Verification items for the finished model (mm, model axes). Face numbers are marked on the shaded views. A direction names the side the tool comes from. Coordinates: 2 decimals unless noted, no trailing zeros. Order: outer loops, then holes, each group sorted by start corner. A loop starts at its lowest first (then second) coordinate and runs counter-clockwise, first axis right, second up. Notation, with made-up numbers: M -10.75,71 L 13.25,71 A22 cw 13.25,82 Z; hole C 86.5,-4 d7. An arc over 180 degrees is marked long. Answer as a JSON object with one key per item and string values. Group by question number.
(1) Mould release check, pull along Y, two halves, no side actions. Record for the marked faces 3, 4 and 5: released by +Y, released by -Y, zero draft, split by the parting line, or undercut.
(2) Gauge pin test, flat ends, axial feed: pin 1 Ø1 at (x, y) = (-3.5, -28) entering from +Z; pin 2 Ø1.5 at (x, z) = (-74.39, -4.15) entering from +Y; pin 3 Ø2 at (x, y) = (-25, -27) entering from -Z. Record the tip position at first contact, or that the pin passes through.
(3) Cross-section at A-A (z = -13). Enter the section's corners in (x, y), plus the area to 3 significant figures.
(4) Material ranges on line 1 (X direction, y = -35, z = -4.15); line 2 (X direction, y = -31.5, z = -13); line 3 (Y direction, x = -78, z = -18), recorded low to high.
(5) Cross-section at C-C (y = -35.75). Count the separate pieces of the cut face and the enclosed holes in it, plus the area to 3 significant figures.
(6) Cross-section at D-D (x = -32.5). Enter the section's corners in (y, z), plus the area to 3 significant figures.
(7) Access from +Z, -Z, +X, -X, +Y, -Y to the whole of each face (thin tool, end or side, straight path). Record for the marked faces 1 and 2.
(8) Cross-section at B-B (z = -19.25). Enter the section's corners in (x, y).
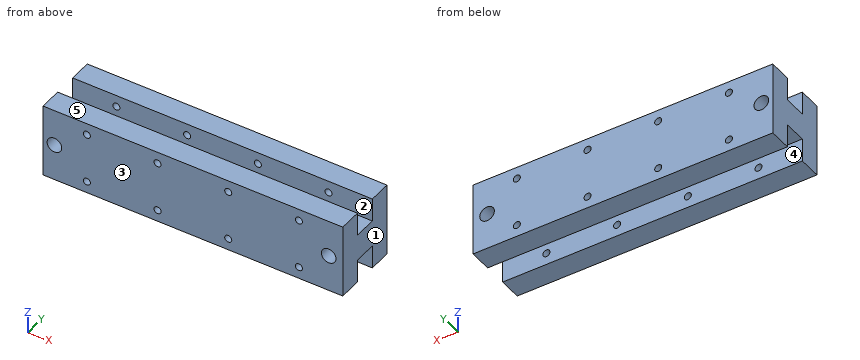
from build123d import *

# Parameters (mm, degrees)
SKETCH4_W                  = 106
SKETCH4_H                  = 24
BOSS_EXTRUDE2_DEPTH        = 13
CUT_EXTRUDE3_START         = -8.3
SKETCH25_W                 = 106
SKETCH25_H                 = 8.1
CUT_EXTRUDE3_DEPTH         = 108.807903902
M3X0_5_TAPPED_HOLE1_D      = 2.5
MIRROR3_START              = -40.65
MIRROR3_OUTLINE_W          = 106
MIRROR3_OUTLINE_H          = 4.7
MIRROR3_DEPTH              = 24
MIRROR3_START_2            = -24.601316976
MIRROR3_2_OUTLINE_W        = 106
MIRROR3_2_OUTLINE_H        = 8.3
MIRROR3_2_OUTLINE_R        = 1.25
MIRROR3_2_DEPTH            = 7.951316976
MIRROR3_3_OUTLINE_W        = 106
MIRROR3_3_OUTLINE_H        = 8.3
MIRROR3_3_OUTLINE_R        = 1.25
MIRROR3_3_DEPTH            = 7.948683024
F_6_0_204_DIAMETER_HOLE1_D = 5.1816


# Read off the part's stored shape, not the designer's step: Mirror3
with BuildPart() as part:
    # Sketch4 → Boss-Extrude2 (new body)
    with BuildSketch(Plane.XY):
        with Locations((-36.891047602, -28.65)):
            Rectangle(SKETCH4_W, SKETCH4_H)
    extrude(amount=-BOSS_EXTRUDE2_DEPTH)

    # Sketch25 → Cut-Extrude3 (cut)
    with BuildSketch(Plane.XY.offset(CUT_EXTRUDE3_START)):
        with Locations((-36.891047602, -28.651316976)):
            Rectangle(SKETCH25_W, SKETCH25_H)
    extrude(amount=CUT_EXTRUDE3_DEPTH, mode=Mode.SUBTRACT)

    # M3x0.5 Tapped Hole1 (through all)
    with Locations(Plane(origin=(-74.390985602, -16.65, -4.15), x_dir=(0, 0, 1), z_dir=(0, 1, 0))):
        with Locations((0, 0), (0, 25), (-0.055677319, 74.999938), (0, 50)):
            Hole(M3X0_5_TAPPED_HOLE1_D / 2)

    # Mirror3 outline → Mirror3 (add)
    with BuildSketch(Plane(origin=(0, 0, 0), x_dir=(1, 0, 0), z_dir=(0, 1, 0)).offset(MIRROR3_START)):
        with Locations((-36.891047602, 15.35)):
            Rectangle(MIRROR3_OUTLINE_W, MIRROR3_OUTLINE_H)
    extrude(amount=MIRROR3_DEPTH)

    # Mirror3 2 outline → Mirror3 2 (add)
    with BuildSketch(Plane(origin=(0, 0, 0), x_dir=(1, 0, 0), z_dir=(0, 1, 0)).offset(MIRROR3_START_2)):
        with Locations((-36.891047602, 21.85)):
            Rectangle(MIRROR3_2_OUTLINE_W, MIRROR3_2_OUTLINE_H)
        with Locations((-74.390985602, 21.85)):
            Circle(MIRROR3_2_OUTLINE_R, mode=Mode.SUBTRACT)
        with Locations((-49.390985602, 21.85)):
            Circle(MIRROR3_2_OUTLINE_R, mode=Mode.SUBTRACT)
        with Locations((-24.390985602, 21.85)):
            Circle(MIRROR3_2_OUTLINE_R, mode=Mode.SUBTRACT)
        with Locations((0.608952398, 21.794322681)):
            Circle(MIRROR3_2_OUTLINE_R, mode=Mode.SUBTRACT)
    extrude(amount=MIRROR3_2_DEPTH)

    # Mirror3 3 outline → Mirror3 3 (add)
    with BuildSketch(Plane(origin=(0, 0, 0), x_dir=(1, 0, 0), z_dir=(0, 1, 0)).offset(MIRROR3_START)):
        with Locations((-36.891047602, 21.85)):
            Rectangle(MIRROR3_3_OUTLINE_W, MIRROR3_3_OUTLINE_H)
        with Locations((-74.390985602, 21.85)):
            Circle(MIRROR3_3_OUTLINE_R, mode=Mode.SUBTRACT)
        with Locations((-49.390985602, 21.85)):
            Circle(MIRROR3_3_OUTLINE_R, mode=Mode.SUBTRACT)
        with Locations((-24.390985602, 21.85)):
            Circle(MIRROR3_3_OUTLINE_R, mode=Mode.SUBTRACT)
        with Locations((0.608952398, 21.794322681)):
            Circle(MIRROR3_3_OUTLINE_R, mode=Mode.SUBTRACT)
    extrude(amount=MIRROR3_3_DEPTH)

    # #6 (0.204) Diameter Hole1 (through all)
    with Locations(Plane(origin=(11.140604923, -40.65, -13), x_dir=(0, 0, -1), z_dir=(0, -1, 0))):
        with Locations((0, 0), (0, -96.994839557)):
            Hole(F_6_0_204_DIAMETER_HOLE1_D / 2)


solid = part.part
Taken from the geometry:
{
 "1": {"face 3": "released by -Y", "face 4": "undercut", "face 5": "zero draft"},
 "2": {"pin 1": "stops at z = -8.3", "pin 2": "passes through", "pin 3": "stops at z = -17.7"},
 "3": {"outline": "M -89.89,-40.65 L -88.45,-40.65 L -88.45,-16.65 L -89.89,-16.65 Z; M -83.26,-40.65 L 8.55,-40.65 L 8.55,-16.65 L -83.26,-16.65 Z; M 13.73,-40.65 L 16.11,-40.65 L 16.11,-16.65 L 13.73,-16.65 Z", "area": "2,300 mm²"},
 "4": {"line 1": "x = -89.89 to -75.64, -73.14 to -50.64, -48.14 to -25.64, -23.14 to -0.64, 1.86 to 16.11", "line 2": "x = -89.89 to -88.45, -83.26 to 8.55, 13.73 to 16.11", "line 3": "y = -40.65 to -32.7, -24.6 to -16.65"},
 "5": {"separate pieces": "1", "enclosed holes": "10", "area": "2,670 mm²"},
 "6": {"outline": "M -40.65,-26 L -32.7,-26 L -32.7,-17.7 L -24.6,-17.7 L -24.6,-26 L -16.65,-26 L -16.65,0 L -24.6,0 L -24.6,-8.3 L -32.7,-8.3 L -32.7,0 L -40.65,0 Z", "area": "490 mm²"},
 "7": {"face 1": "+Z, -Z, +X, +Y, -Y", "face 2": "+Z, +X, -X"},
 "8": {"outline": "M -89.89,-40.65 L 16.11,-40.65 L 16.11,-32.7 L -89.89,-32.7 Z; M -89.89,-24.6 L 16.11,-24.6 L 16.11,-16.65 L -89.89,-16.65 Z"}
}
